Model file for the job. Use its own axes, mm. A direction names the side the tool comes from. Coordinates: 2 decimals unless noted, no trailing zeros. Write each loop counter-clockwise with the first axis right and the second up, starting at its lowest first coordinate (ties: lowest second). Pieces come first, ordered by that corner, then holes. Notation, with made-up numbers: M 25.25,-36 L 38.25,-36 A24 ccw 38.25,-10 Z; hole C 55,39 d7. An arc over 180 degrees is marked long. Answer in a Markdown table with one row per item. Add a question column.
```python
from build123d import *

# Parameters (mm, degrees)
SKETCH_1_R          = 11
EXTRUDE_1_DEPTH     = 2
SKETCH_2_R          = 5
EXTRUDE_2_DEPTH     = 10
SKETCH_3_R          = 2.5
CUT_EXTRUDE_1_DEPTH = 10
HOLE_WIZARD_1_D     = 3
FILLET_1_R          = 0.5


with BuildPart() as part:
    # 草图1 → 凸台-拉伸1 (new body)
    with BuildSketch(Plane(origin=(0, 0, 0), x_dir=(1, 0, 0), z_dir=(0, 1, 0))):
        with Locations(Location((0, 0, 0), (0, 0, 270))):
            Circle(SKETCH_1_R)
    extrude(amount=EXTRUDE_1_DEPTH)

    # 草图2 → 凸台-拉伸2 (add)
    with BuildSketch(Plane(origin=(0, 2, 0), x_dir=(1, 0, 0), z_dir=(0, 1, 0))):
        with Locations(Location((0, 0, 0), (0, 0, 270))):
            Circle(SKETCH_2_R)
    extrude(amount=EXTRUDE_2_DEPTH)

    # 草图3 → 切除-拉伸1 (cut)
    with BuildSketch(Plane(origin=(0, 12, 0), x_dir=(1, 0, 0), z_dir=(0, 1, 0))):
        with Locations(Location((0, 0, 0), (0, 0, 270))):
            Circle(SKETCH_3_R)
    extrude(amount=-CUT_EXTRUDE_1_DEPTH, mode=Mode.SUBTRACT)

    # 孔1 (through all)
    with Locations(Plane(origin=(0, 2, 0), x_dir=(1, 0, 0), z_dir=(0, 1, 0))):
        with Locations((0, 8), (8, 0), (0, -8), (-8, 0)):
            Hole(HOLE_WIZARD_1_D / 2)

    # 圆角1
    fillet_1_edges = [part.edges().sort_by_distance(p)[0] for p in [
        (0, 2, -11),
        (0, 12, -5),
    ]]
    fillet(fillet_1_edges, radius=FILLET_1_R)


solid = part.part
```
1) Slice it at B-B (y = 6.5). Give the cut face in (x, z).
2) Flat gauge pins, fed straight in: pin 1 Ø3 at (x, y) = (4.5, 5.5) entering from -Z; pin 2 Ø1.5 at (x, z) = (-3.5, -8.5) entering from +Y; pin 3 Ø1.5 at (y, z) = (6.5, -2.5) entering from -X. Where does each tip first touch, or does it go through?
3) Two-plate mould, pull along Z, no slides. Class faces 1 (the face through (-6.5, 0.99, -0.07)), 2 (the face through (-10.74, 0.74, -2.38)), 3 (the face through (0, 0, 0)): released by +Z, released by -Z, zero draft, split by the parting line, or undercut.
4) Which spindle directions (+Z, -Z, +X, -X, +Y, -Y) get a long thin tool onto all of the face, cutting with end or side? Do faces 4 (the face through (0.325, 0.986, 9.464)), 5 (the face through (0, 2, 0)). Say none if no direction does.
5) Drill centre lines: probe 1 along X at (y, z) = (6, 0); probe 2 along Y at (x, z) = (6.5, -1.75); probe 3 along Z at (x, y) = (1, 6). Where is each one in solid material? Low to high.
6) Slice it at A-A (z = 0). Give the cut face in (x, y).
Ans:
| question | item | result |
|---|---|---|
| 1 | outline | C 0,0 d10; hole C 0,0 d5 |
| 2 | pin 1 | stops at z = -4 |
| 2 | pin 2 | stops at y = 2 |
| 2 | pin 3 | stops at x = -4.68 |
| 3 | face 1 | undercut |
| 3 | face 2 | split by the parting line |
| 3 | face 3 | zero draft |
| 4 | face 4 | +Y, -Y |
| 4 | face 5 | +Y |
| 5 | probe 1 | x = -5 to -2.5, 2.5 to 5 |
| 5 | probe 2 | y = 0 to 2 |
| 5 | probe 3 | z = -4.9 to -2.29, 2.29 to 4.9 |
| 6 | outline | M -11,0 L -9.5,0 L -9.5,2 L -10.5,2 A0.5 ccw -11,1.5 Z; M -6.5,0 L 6.5,0 L 6.5,2 L 5,2 L 5,11.5 A0.5 ccw 4.5,12 L 2.5,12 L 2.5,2 L -2.5,2 L -2.5,12 L -4.5,12 A0.5 ccw -5,11.5 L -5,2 L -6.5,2 Z; M 9.5,0 L 11,0 L 11,1.5 A0.5 ccw 10.5,2 L 9.5,2 Z |
